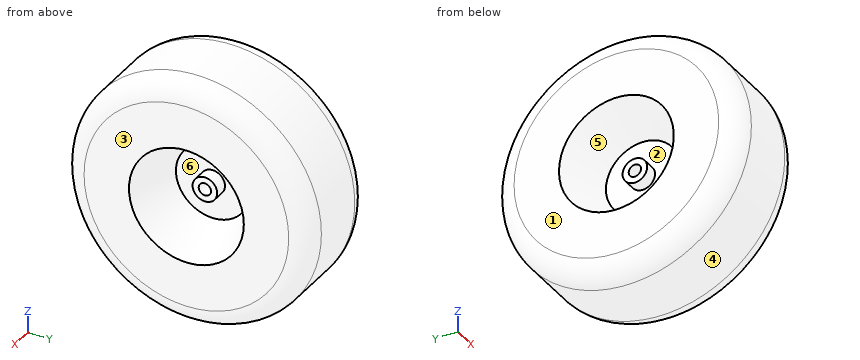
```python
from build123d import *


with BuildPart() as part:
    # Sketch1 → Revolve1 (revolve)
    with BuildSketch(Plane.XY):
        with BuildLine():
            Line((-26.9875, 9.525), (26.9875, 9.525))
            Line((26.9875, 9.525), (26.9875, 19.05))
            Line((26.9875, 19.05), (6.112639692, 19.05))
            Line((6.112639692, 19.05), (6.112639692, 56.974587415))
            Line((6.112639692, 56.974587415), (76.2, 88.9))
            Line((76.2, 88.9), (76.2, 158.372961578))
            ThreePointArc((76.2, 158.372961578), (66.923900362, 180.957937381), (44.45, 190.5))
            Line((44.45, 190.5), (-44.45, 190.5))
            ThreePointArc((-44.45, 190.5), (-66.923900362, 180.957937381), (-76.2, 158.372961578))
            Line((-76.2, 158.372961578), (-76.2, 88.9))
            Line((-76.2, 88.9), (-6.112639692, 56.974587415))
            Line((-6.112639692, 56.974587415), (-6.112639692, 19.05))
            Line((-6.112639692, 19.05), (-26.9875, 19.05))
            Line((-26.9875, 19.05), (-26.9875, 9.525))
        make_face()
    revolve(axis=Axis((-76.2, 0, 0), (1, 0, 0)))


solid = part.part
```
Work out the finished part from the listing and answer in its coordinate system (mm). Face numbers are marked on the shaded views. A direction names the side the tool comes from. Round coordinates to 2 decimals unless told otherwise and drop trailing zeros. Write each loop counter-clockwise with the first axis right and the second up, starting at its lowest first coordinate (ties: lowest second). Pieces come first, ordered by that corner, then holes. Notation, with made-up numbers: (87.5, -23.75) - (108.5, -23.75) arc R30 cw to (108.5, 2.25) - close; hole circle Ø11 at (36.25, -37.5). An arc over 180 degrees is marked (long way). Return JSON: item names as keys, results as strings. Group by question number.
Q1. The part is cut by section C-C on x = -53. Write down the section's boundary in (y, z), then the cut area to 3 significant figures.
Q2. Each of these flat-tipped pins is pushed along its axis until it touches: pin 1 Ø2 at (x, z) = (46, -68.5) entering from +Y; pin 2 Ø6 at (x, z) = (16.5, -18.5) entering from +Y; pin 3 Ø11.5 at (y, z) = (9, 3.5) entering from -X. Where does it stop, or does it pass through?
Q3. For the marked faces 1 and 2, determine the directions among +Z, -Z, +X, -X, +Y, -Y from which every point of the face is accessible in a straight line to the end or side of a thin tool.
Q4. The part is cut by section D-D on x = -0.5. Write down the section's boundary in (y, z) (3 decimals), then the cut area to 3 significant figures.
Q5. The mould has two halves that part along Y. Classify the marked faces 3, 4, 5 and 6: released by +Y, released by -Y, zero draft, split by the parting line, or undercut.
Q6. Find the intervals of material crossed by L1, parallel to Z at x = 11, y = 0 (3 decimals); L2, parallel to Z at x = -9, y = 0 (3 decimals); L3, parallel to X at y = 79.5, z = 139, in increasing order.
Solved:
{
 "1": {"outline": "circle Ø378.47 at (0, 0); hole circle Ø156.66 at (0, 0)", "area": "93,200 mm²"},
 "2": {"pin 1": "y = 178.09", "pin 2": "y = 189.87", "pin 3": "x = -26.99"},
 "3": {"face 1": "+Z, -Z, -X, +Y, -Y", "face 2": "-X"},
 "4": {"outline": "circle Ø381 at (0, 0); hole circle Ø19.05 at (0, 0)", "area": "114,000 mm²"},
 "5": {"face 3": "zero draft", "face 4": "split by the parting line", "face 5": "undercut", "face 6": "undercut"},
 "6": {"L1": "-190.5 to -59.201, -19.05 to -9.525, 9.525 to 19.05, 59.201 to 190.5", "L2": "-190.5 to -58.29, -19.05 to -9.525, 9.525 to 19.05, 58.29 to 190.5", "L3": "-76.15 to 76.15"}
}
